from build123d import *

# Parameters (mm, degrees)
F0_W     = 3.81
F0_H     = 25.4
F1_DEPTH = 12.7
F2_R     = 3.81
F3_DEPTH = 7.62
F5_DEPTH = 7.62
F6_DEPTH = 7.62
F7_R     = 1.61925
F8_DEPTH = 25.4


with BuildPart() as f1:
    # F0 (on Front) → F1 (new body)
    with BuildSketch(Plane.XZ):
        Rectangle(F0_W, F0_H)
    extrude(amount=F1_DEPTH)

    # F2 (on face) → F3 (join)
    with BuildSketch(Plane.XY.offset(12.7)):
        with Locations((1.905, 0)):
            Circle(F2_R)
    extrude(amount=-F3_DEPTH)

    # F2 (on face) → F5 (join)
    with BuildSketch(Plane.XY.offset(12.7)):
        with Locations((1.905, 0)):
            Circle(F2_R)
    extrude(amount=-F5_DEPTH)

    # F4 (on face) → F6 (join)
    with BuildSketch(Plane(origin=(0, 0, -12.7), x_dir=(1, 0, 0), z_dir=(0, 0, -1))):
        with BuildLine():
            Line((1.905, 0), (-1.905, 0))
            ThreePointArc((-1.905, 0), (1.905, -3.81), (5.715, 0))
            ThreePointArc((5.715, 0), (4.5990768363, 2.6940768363), (1.905, 3.81))
            Line((1.905, 3.81), (1.905, 0))
        make_face()
    extrude(amount=-F6_DEPTH)

    # F7 (on face) → F8 (cut)
    with BuildSketch(Plane.XY.offset(12.7)):
        with Locations((1.905, 0)):
            Circle(F7_R)
    extrude(amount=-F8_DEPTH, mode=Mode.SUBTRACT)


solid = f1.part
Work out the finished part from the listing and answer in its coordinate system (mm). A direction names the side the tool comes from. Give positions to 0.01 mm unless a question says otherwise; leave off trailing zeros. Order: outer loops, then holes, each group sorted by start corner. A loop starts at its lowest first (then second) coordinate and runs counter-clockwise, first axis right, second up. Notation, with made-up numbers: (79, 65.25) - (96, 65.25) arc R11 cw to (96, 79.25) - close; hole circle Ø10 at (63.25, -30). An arc over 180 degrees is marked (long way). Answer as CSV lines item,"result". Start each with the question number.
Q1. For faces 5 (the face through (4.69, 2.6, 8.94)), 6 (the face through (4, 1, -5.08)), determine the directions among +Z, -Z, +X, -X, +Y, -Y from which every point of the face is accessible in a straight line to the end or side of a thin tool.
Q2. The part is cut by section B-B (y = -0.5). Write down the section's boundary in (x, z) (3 decimals).
Q3. Find the intervals of material crossed by L1, parallel to Z at x = 4, y = 0.5; L2, parallel to X at y = -4.5, z = -8.25 (3 decimals); L3, parallel to Y at x = -0.25, z = -0.5, in increasing order. Write a range as [from, to].
Q4. The part is cut by section A-A (z = -6). Write down the section's boundary in (x, y) (1 decimal).
Q5. Given pin 1 Ø4 at (x, z) = (2, -1) entering from +Y; pin 2 Ø3 at (x, y) = (1.905, 0) entering from -Z; pin 3 Ø1 at (y, z) = (-7, 5) entering from +X (3 decimals); pin 4 Ø8 at (y, z) = (-6, 2.5) entering from +X, each flat-ended and moving along its own axis, determine where each tip first touches the part or whether it passes through.
Q6. The part is cut by section C-C (x = 2.25). Write down the section's boundary in (y, z).
Q7. The mould has two halves that part along Z. Classify faces 1 (the face through (1, -5, -12.7)), 2 (the face through (0, -12.7, 0)), 3 (the face through (-1, 0, 0)), 4 (the face through (4, 1, 5.08)): +Z half, -Z half, draft (parallel to the pull), parting line (faces both ways), or undercut.
Q8. The part is cut by section D-D (y = 1.25). Write down the section's boundary in (x, z).
Check result:
1,face 5,"+Z, -Z"
1,face 6,"+X, +Y"
2,outline,"(-1.905, -12.7) - (0.365, -12.7) - (0.365, 12.7) - (-1.905, 12.7) - close; (3.445, -12.7) - (5.682, -12.7) - (5.682, -5.08) - (3.445, -5.08) - close; (3.445, 5.08) - (5.682, 5.08) - (5.682, 12.7) - (3.445, 12.7) - close"
3,L1,"z = [-12.7, -5.08], [5.08, 12.7]"
3,L2,"x = [-1.905, 1.905]"
3,L3,"y = [-12.7, 0]"
4,outline,"(-1.9, -12.7) - (1.9, -12.7) - (1.9, -3.8) arc R3.8 ccw (long way) to (-1.9, 0) - close; hole circle Ø3.2 at (1.9, 0)"
5,pin 1,"stops at y = 0"
5,pin 2,"passes through"
5,pin 3,"stops at x = 1.905"
5,pin 4,"stops at x = 4.32"
6,outline,"(-3.79, -12.7) - (-1.58, -12.7) - (-1.58, -5.08) - (-3.79, -5.08) - close; (-3.79, 5.08) - (-1.58, 5.08) - (-1.58, 12.7) - (-3.79, 12.7) - close; (1.58, -12.7) - (3.79, -12.7) - (3.79, -5.08) - (1.58, -5.08) - close; (1.58, 5.08) - (3.79, 5.08) - (3.79, 12.7) - (1.58, 12.7) - close"
7,face 1,"-Z half"
7,face 2,"draft"
7,face 3,"undercut"
7,face 4,"undercut"
8,outline,"(-1.69, -12.7) - (0.88, -12.7) - (0.88, -5.08) - (-1.69, -5.08) - close; (-1.69, 5.08) - (0.88, 5.08) - (0.88, 12.7) - (-1.69, 12.7) - close; (2.93, -12.7) - (5.5, -12.7) - (5.5, -5.08) - (2.93, -5.08) - close; (2.93, 5.08) - (5.5, 5.08) - (5.5, 12.7) - (2.93, 12.7) - close"
